from build123d import *

# Parameters (mm, degrees)
F0_W      = 203.2
F0_H      = 152.4
F2_DEPTH  = 152.4
F3_W      = 88.9
F3_H      = 139.7
F4_DEPTH  = 12.7
F5_R      = 6.35
F6_DEPTH  = 127
F1_R      = 44.45
F8_DEPTH  = 101.6
F9_R      = 5.08
F10_W     = 127
F10_H     = 139.7
F11_DEPTH = 101.6
F12_W     = 193.04
F12_H     = 142.24
F12_W_2   = 88.9
F12_H_2   = 139.7
F12_R     = 44.45
F12_R_2   = 6.35
F14_W     = 88.9
F14_H     = 139.7
F14_W_2   = 312.5441968441
F14_H_2   = 209.9168300629
F15_DEPTH = 29.21
F13_W     = 76.2
F13_H     = 127
F16_DEPTH = 152.4
F17_W     = 88.9
F17_H     = 127
F18_DEPTH = 253.619
F19_W     = 12.7
F19_H     = 38.596359849
F19_H_2   = 95.0815806389
F19_H_3   = 79.8769908249
F19_H_4   = 69.7309503555
F19_H_5   = 88.4333456159
F20_DEPTH = 6.35
F21_W     = 76.2
F21_H     = 12.7
F22_DEPTH = 6.35
F23_W     = 12.7
F23_H     = 76.2
F23_H_2   = 86.7299305499
F23_H_3   = 88.9
F24_DEPTH = 6.35
F25_W     = 12.7
F25_H     = 12.7
F25_H_2   = 12.4177324921
F25_H_3   = 127
F25_W_2   = 2.5730909735
F25_H_4   = 12.9822675079
F26_DEPTH = 12.7


with BuildPart() as f2:
    # F0 (on Front) → F2 (new body)
    with BuildSketch(Plane.XZ):
        Rectangle(F0_W, F0_H)
    extrude(amount=F2_DEPTH)

    # F3 (on Front) → F4 (cut)
    with BuildSketch(Plane.XZ):
        with Locations((-50.6012091197, -0.215793407)):
            Rectangle(F3_W, F3_H)
    extrude(amount=F4_DEPTH, mode=Mode.SUBTRACT)

    # F5 (on face) → F6 (cut)
    with BuildSketch(Plane(origin=(0, -12.7, 0), x_dir=(-1, 0, 0), z_dir=(0, 1, 0))):
        with Locations((19.2305770945, 52.8817098261)):
            Circle(F5_R)
        with Locations((19.2305770945, 31.2917098261)):
            Circle(F5_R)
        with Locations((19.2305770945, 9.7017098261)):
            Circle(F5_R)
        with Locations((19.2305770945, -11.8882901739)):
            Circle(F5_R)
        with Locations((19.2305770945, -33.4782901739)):
            Circle(F5_R)
        with Locations((19.2305770945, -55.0682901739)):
            Circle(F5_R)
        with Locations((40.8205770945, 52.8817098261)):
            Circle(F5_R)
        with Locations((40.8205770945, 31.2917098261)):
            Circle(F5_R)
        with Locations((40.8205770945, 9.7017098261)):
            Circle(F5_R)
        with Locations((40.8205770945, -11.8882901739)):
            Circle(F5_R)
        with Locations((40.8205770945, -33.4782901739)):
            Circle(F5_R)
        with Locations((40.8205770945, -55.0682901739)):
            Circle(F5_R)
        with Locations((62.4105770945, 52.8817098261)):
            Circle(F5_R)
        with Locations((62.4105770945, 31.2917098261)):
            Circle(F5_R)
        with Locations((62.4105770945, 9.7017098261)):
            Circle(F5_R)
        with Locations((62.4105770945, -11.8882901739)):
            Circle(F5_R)
        with Locations((62.4105770945, -33.4782901739)):
            Circle(F5_R)
        with Locations((62.4105770945, -55.0682901739)):
            Circle(F5_R)
        with Locations((84.0005770945, 52.8817098261)):
            Circle(F5_R)
        with Locations((84.0005770945, 31.2917098261)):
            Circle(F5_R)
        with Locations((84.0005770945, 9.7017098261)):
            Circle(F5_R)
        with Locations((84.0005770945, -11.8882901739)):
            Circle(F5_R)
        with Locations((84.0005770945, -33.4782901739)):
            Circle(F5_R)
        with Locations((84.0005770945, -55.0682901739)):
            Circle(F5_R)
    extrude(amount=-F6_DEPTH, mode=Mode.SUBTRACT)

    # F1 (on face) → F8 (cut)
    with BuildSketch(Plane.XZ):
        with Locations((48.0613298714, 0)):
            Circle(F1_R)
    extrude(amount=F8_DEPTH, mode=Mode.SUBTRACT)

    # F9
    f9_edges = [f2.edges().sort_by_distance(p)[0] for p in [
        (0, 0, 76.2),
        (101.6, 0, 0),
        (0, 0, -76.2),
        (-101.6, 0, 0),
        (-101.6, -76.2, -76.2),
        (101.6, -76.2, -76.2),
        (101.6, -76.2, 76.2),
        (-101.6, -76.2, 76.2),
    ]]
    fillet(f9_edges, radius=F9_R)

    # F10 (on face) → F11 (cut)
    with BuildSketch(Plane(origin=(-101.6, 0, 0), x_dir=(0, -1, 0), z_dir=(-1, 0, 0))):
        with Locations((76.9326984882, 0)):
            Rectangle(F10_W, F10_H)
    extrude(amount=-F11_DEPTH, mode=Mode.SUBTRACT)

    # F12 (on face) + F14 (on face) → F15 (cut)
    with BuildSketch(Plane(origin=(0, 0, 0), x_dir=(-1, 0, 0), z_dir=(0, 1, 0))):
        Rectangle(F12_W, F12_H)
        with Locations((50.6012091197, -0.215793407)):
            Rectangle(F12_W_2, F12_H_2, mode=Mode.SUBTRACT)
        with Locations((-48.0613298714, 0)):
            Circle(F12_R, mode=Mode.SUBTRACT)
        with Locations((-87.3994901776, 62.0860531926)):
            Circle(F12_R_2, mode=Mode.SUBTRACT)
    with BuildSketch(Plane(origin=(0, 0, 0), x_dir=(-1, 0, 0), z_dir=(0, 1, 0))):
        with Locations((50.6012091197, -0.215793407)):
            Rectangle(F14_W, F14_H)
        Rectangle(F14_W_2, F14_H_2)
    extrude(amount=-F15_DEPTH, mode=Mode.SUBTRACT)

    # F13 (on face) → F16 (cut)
    with BuildSketch(Plane(origin=(0, 0, -76.2), x_dir=(1, 0, 0), z_dir=(0, 0, -1))):
        with Locations((-52.4439588189, 78.7642598152)):
            Rectangle(F13_W, F13_H)
    extrude(amount=-F16_DEPTH, mode=Mode.SUBTRACT)

    # F17 (on Top) → F18 (cut, symmetric)
    with BuildSketch(Plane.XY):
        with Locations((40.8431477845, -78.819476068)):
            Rectangle(F17_W, F17_H)
    extrude(amount=F18_DEPTH, both=True, mode=Mode.SUBTRACT)

    # F19 (on face) → F20 (join)
    with BuildSketch(Plane.XY.offset(76.2)):
        with Locations((78.9431477845, -123.0212961435)):
            Rectangle(F19_W, F19_H)
        Polygon((59.8931477845, -142.319476068), (59.8931477845, -56.6326193511), (59.8931477845, -28.019476068), (47.1931477845, -28.019476068), (47.1931477845, -47.2378954291), (47.1931477845, -142.319476068), align=None)
        Polygon((72.5931477845, -142.319476068), (72.5931477845, -103.723116219), (72.5931477845, -56.6326193511), (59.8931477845, -56.6326193511), (59.8931477845, -142.319476068), align=None)
        with Locations((40.8431477845, -94.7786857486)):
            Rectangle(F19_W, F19_H_2)
        Polygon((21.7931477845, -62.4424852431), (21.7931477845, -142.319476068), (34.4931477845, -142.319476068), (34.4931477845, -47.2378954291), (34.4931477845, 16.430523932), (21.7931477845, 16.430523932), align=None)
        with Locations((15.4431477845, -102.3809806556)):
            Rectangle(F19_W, F19_H_3)
        with Locations((-20.6939588189, -107.3987846375)):
            Rectangle(F19_W, F19_H_4)
        Polygon((-39.7439588189, -53.8309141994), (-39.7439588189, -142.2642598152), (-27.0439588189, -142.2642598152), (-27.0439588189, -72.5333094597), (-27.0439588189, -27.9642598152), (-39.7439588189, -27.9642598152), align=None)
        with Locations((-46.0939588189, -98.0475870073)):
            Rectangle(F19_W, F19_H_5)
        Polygon((-65.1439588189, -40.6642598152), (-65.1439588189, -142.2642598152), (-52.4439588189, -142.2642598152), (-52.4439588189, -53.8309141994), (-52.4439588189, 10.1357401848), (-65.1439588189, 10.1357401848), align=None)
        Polygon((-77.8439588189, -91.4642598152), (-77.8439588189, -142.2642598152), (-65.1439588189, -142.2642598152), (-65.1439588189, -40.6642598152), (-77.8439588189, -40.6642598152), align=None)
        Polygon((-3.6068522155, -28.019476068), (-3.6068522155, -29.21), (-3.6068522155, -142.319476068), (9.0931477845, -142.319476068), (9.0931477845, -62.4424852431), (9.0931477845, -28.019476068), align=None)
    extrude(amount=-F20_DEPTH)

    # F21 (on face) → F22 (join)
    with BuildSketch(Plane(origin=(-101.6, 0, 0), x_dir=(0, -1, 0), z_dir=(-1, 0, 0))):
        Polygon((13.4326984882, -57.15), (13.4326984882, -69.85), (140.4326984882, -69.85), (140.4326984882, -57.15), (64.2326984882, -57.15), align=None)
        with Locations((102.3326984882, -50.8)):
            Rectangle(F21_W, F21_H)
        Polygon((26.1326984882, -25.4), (26.1326984882, -38.1), (140.4326984882, -38.1), (140.4326984882, -25.4), (64.2326984882, -25.4), align=None)
        with Locations((102.3326984882, -19.05)):
            Rectangle(F21_W, F21_H)
        Polygon((64.2326984882, -12.7), (140.4326984882, -12.7), (140.4326984882, 0), (41.91, 0), (41.91, -12.7), align=None)
        Polygon((41.91, 0), (140.4326984882, 0), (140.4326984882, 12.7), (38.8326984882, 12.7), (38.8326984882, 0), align=None)
        Polygon((13.4326984882, 31.75), (13.4326984882, 19.05), (140.4326984882, 19.05), (140.4326984882, 31.75), (26.1326984882, 31.75), align=None)
        Polygon((26.1326984882, 31.75), (140.4326984882, 31.75), (140.4326984882, 44.45), (64.2326984882, 44.45), (26.1326984882, 44.45), align=None)
        with Locations((102.3326984882, 50.8)):
            Rectangle(F21_W, F21_H)
        Polygon((64.2326984882, 57.15), (140.4326984882, 57.15), (140.4326984882, 69.85), (26.1326984882, 69.85), (26.1326984882, 57.15), align=None)
    extrude(amount=-F22_DEPTH)

    # F23 (on face) → F24 (join)
    with BuildSketch(Plane(origin=(0, 0, -76.2), x_dir=(1, 0, 0), z_dir=(0, 0, -1))):
        with Locations((78.9431477845, 104.219476068)):
            Rectangle(F23_W, F23_H)
        with Locations((2.7431477845, 98.9545107931)):
            Rectangle(F23_W, F23_H_2)
        with Locations((-20.6939588189, 97.8142598152)):
            Rectangle(F23_W, F23_H_3)
        Polygon((72.5931477845, 28.019476068), (72.5931477845, 66.119476068), (72.5931477845, 142.319476068), (59.8931477845, 142.319476068), (59.8931477845, 28.019476068), align=None)
        Polygon((59.8931477845, 28.019476068), (59.8931477845, 142.319476068), (47.1931477845, 142.319476068), (47.1931477845, 53.419476068), (47.1931477845, 15.319476068), (59.8931477845, 15.319476068), align=None)
        with Locations((40.8431477845, 97.869476068)):
            Rectangle(F23_W, F23_H_3)
        Polygon((34.4931477845, 53.419476068), (34.4931477845, 142.319476068), (21.7931477845, 142.319476068), (21.7931477845, 40.719476068), (21.7931477845, 28.019476068), (34.4931477845, 28.019476068), align=None)
        Polygon((21.7931477845, 40.719476068), (21.7931477845, 142.319476068), (9.0931477845, 142.319476068), (9.0931477845, 55.5895455182), (9.0931477845, 40.719476068), align=None)
        Polygon((-27.0439588189, 142.2642598152), (-39.7439588189, 142.2642598152), (-39.7439588189, 34.2246964574), (-27.0439588189, 34.2246964574), (-27.0439588189, 53.3642598152), align=None)
        Polygon((-39.7439588189, 142.2642598152), (-52.4439588189, 142.2642598152), (-52.4439588189, 27.9642598152), (-39.7439588189, 27.9642598152), (-39.7439588189, 34.2246964574), align=None)
        Polygon((-52.4439588189, 142.2642598152), (-65.1439588189, 142.2642598152), (-65.1439588189, 66.0642598152), (-65.1439588189, 2.5642598152), (-52.4439588189, 2.5642598152), (-52.4439588189, 27.9642598152), align=None)
        with Locations((-71.4939588189, 104.1642598152)):
            Rectangle(F23_W, F23_H)
        Polygon((-90.5439588189, 142.2642598152), (-90.5439588189, 29.21), (-90.5439588189, 27.9642598152), (-77.8439588189, 27.9642598152), (-77.8439588189, 66.0642598152), (-77.8439588189, 142.2642598152), align=None)
    extrude(amount=-F24_DEPTH)

    # F25 (on face) → F26 (join)
    with BuildSketch(Plane.XZ.offset(152.4)):
        Polygon((85.4586139321, 64.0224360317), (61.2050529242, 64.0224360317), (48.5050529242, 64.0224360317), (7.57732118, 64.0224360317), (-5.12267882, 64.0224360317), (-26.6723212183, 64.0224360317), (-39.3723212183, 64.0224360317), (-102.4682950944, 64.0224360317), (-102.4682950944, 44.3732525826), (-89.7682950944, 44.3732525826), (-89.7682950944, 31.6732525826), (-102.4682950944, 31.6732525826), (-102.4682950944, -25.3421988666), (-89.7682950944, -25.3421988666), (-89.7682950944, -38.0421988666), (-102.4682950944, -38.0421988666), (-102.4682950944, -62.9775639683), (-89.4405841827, -62.9775639683), (-76.7405841827, -62.9775639683), (-52.6970252395, -62.9775639683), (-39.9970252395, -62.9775639683), (22.5620511919, -62.9775639683), (35.2620511919, -62.9775639683), (59.3553744256, -62.9775639683), (72.0553744256, -62.9775639683), (85.4586139321, -62.9775639683), align=None)
        with Locations((54.8550529242, 70.3724360317)):
            Rectangle(F25_W, F25_H)
        with Locations((91.8086139321, 70.2313022777)):
            Rectangle(F25_W, F25_H_2)
        with Locations((91.8086139321, 0.5224360317)):
            Rectangle(F25_W, F25_H_3)
        with Locations((1.22732118, 70.3724360317)):
            Rectangle(F25_W, F25_H)
        with Locations((99.4451594189, 0.5224360317)):
            Rectangle(F25_W_2, F25_H_3)
        with Locations((91.8086139321, -69.4686977223)):
            Rectangle(F25_W, F25_H_4)
        with Locations((65.7053744256, -69.3275639683)):
            Rectangle(F25_W, F25_H)
        with Locations((-33.0223212183, 70.3724360317)):
            Rectangle(F25_W, F25_H)
        with Locations((28.9120511919, -69.3275639683)):
            Rectangle(F25_W, F25_H)
        with Locations((-96.1182950944, 38.0232525826)):
            Rectangle(F25_W, F25_H)
        with Locations((-46.3470252395, -69.3275639683)):
            Rectangle(F25_W, F25_H)
        with Locations((-96.1182950944, -31.6921988666)):
            Rectangle(F25_W, F25_H)
        with Locations((-83.0905841827, -69.3275639683)):
            Rectangle(F25_W, F25_H)
    extrude(amount=F26_DEPTH)


solid = f2.part
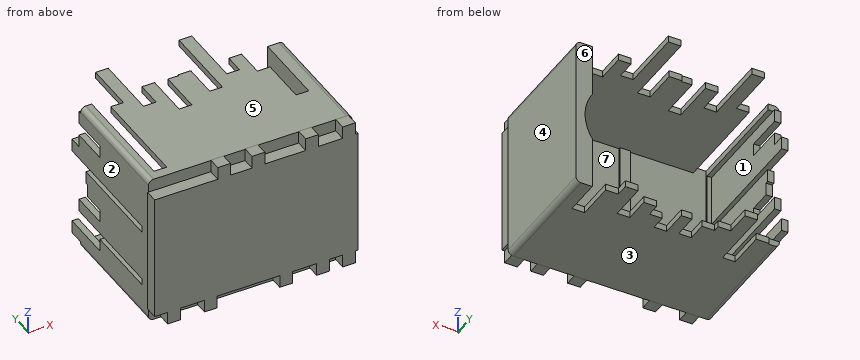
Geometry check sheet. Reference: the model listing, model coordinates, mm. Face numbers are marked on the shaded views. A direction names the side the tool comes from. Give positions to 0.01 mm unless a question says otherwise; leave off trailing zeros. Order: outer loops, then holes, each group sorted by start corner. A loop starts at its lowest first (then second) coordinate and runs counter-clockwise, first axis right, second up.
1) Cross-section at B-B (y = -135.5). Record the boundary of the cut face in (x, z).
Results are:
outline: (-101.6, -71.12) arc R5.08 ccw to (-96.52, -76.2) - (96.52, -76.2) arc R5.08 ccw to (101.6, -71.12) - (101.6, 71.12) arc R5.08 ccw to (96.52, 76.2) - (-77.84, 76.2) - (-77.84, 69.85) - (85.29, 69.85) - (85.29, -69.85) - (-95.25, -69.85) - (-95.25, -44.45) - (-101.6, -44.45) - close; (-101.6, -38.1) - (-95.25, -38.1) - (-95.25, 12.7) - (-101.6, 12.7) - close; (-101.6, 19.05) - (-95.25, 19.05) - (-95.25, 69.85) - (-90.54, 69.85) - (-90.54, 76.2) - (-96.52, 76.2) arc R5.08 ccw to (-101.6, 71.12) - close
2) Material ranges on probe 1 along X at (y, z) = (-65, 70.5); probe 2 along Z at (x, y) = (24, -87); probe 3 along X at (y, z) = (-107, 0.5), recorded low to high.
Results are:
probe 1: x = -101.6 to -90.54, -77.84 to -27.04, -14.34 to 72.59, 85.29 to 101.6
probe 2: z = -76.2 to -69.85, 69.85 to 76.2
probe 3: x = -101.6 to -95.25, 85.29 to 101.6
3) Cross-section at C-C (x = 56). Record the boundary of the cut face in (y, z).
Results are:
outline: (-165.1, -62.98) - (-152.4, -62.98) - (-152.4, -76.2) - (-15.32, -76.2) - (-15.32, -69.85) - (-142.32, -69.85) - (-142.32, 69.85) - (-28.02, 69.85) - (-28.02, 76.2) - (-152.4, 76.2) - (-152.4, 76.72) - (-165.1, 76.72) - close
4) Tool access check on the marked faces 5, 6 and 7. Record the directions out of +Z, -Z, +X, -X, +Y, -Y that give a thin tool (end or side, any length) a straight path to the whole face; none if there is none.
Results are:
face 5: +Z, +X, -X, +Y
face 6: +Z, -Z, +X, +Y
face 7: +Y
5) Draft check along X on the marked faces 1, 2, 3 and 4. Enter one of: released by +X, released by -X, zero draft, split by the parting line, or undercut.
Results are:
face 1: undercut
face 2: released by -X
face 3: zero draft
face 4: released by +X
6) Gauge pin test, flat ends, axial feed: pin 1 (5 mm diameter, centred on x = -97.5, z = 49, fed in from +Y); pin 2 (6 mm diameter, centred on x = -66.5, z = -19.5, fed in from +Y); pin 3 (13.5 mm diameter, centred on y = -156, z = 71, fed in from -X); pin 4 (5 mm diameter, centred on x = -99, y = -72, fed in from -Z). Record the tip position at first contact, or that the pin passes through.
Results are:
pin 1: stops at y = -64.23
pin 2: stops at y = -142.26
pin 3: stops at x = -101.6
pin 4: stops at z = -76.2
7) Cross-section at A-A (y = -21). Record the boundary of the cut face in (x, z), then the cut area to 3 significant figures.
Results are:
outline: (-101.6, -69.85) - (-95.25, -69.85) - (-95.25, -57.15) - (-101.6, -57.15) - close; (-101.6, 19.05) - (-95.25, 19.05) - (-95.25, 31.75) - (-101.6, 31.75) - close; (-65.14, -76.2) - (-52.44, -76.2) - (-52.44, -69.85) - (-65.14, -69.85) - close; (-65.14, 69.85) - (-52.44, 69.85) - (-52.44, 76.2) - (-65.14, 76.2) - close; (21.79, 69.85) - (34.49, 69.85) - (34.49, 76.2) - (21.79, 76.2) - close; (47.19, -76.2) - (59.89, -76.2) - (59.89, -69.85) - (47.19, -69.85) - close
area: 484 mm2
8) Cross-section at D-D (z = 40.5). Record the boundary of the cut face in (x, y), then the cut area to 3 significant figures.
Results are:
outline: (-102.47, -165.1) - (100.73, -165.1) - (100.73, -152.4) - (101.6, -152.4) - (101.6, -29.21) - (85.29, -29.21) - (85.29, -142.32) - (-3.61, -142.32) - (-3.61, -140.43) - (-14.34, -140.43) - (-14.34, -142.26) - (-90.54, -142.26) - (-90.54, -140.43) - (-95.25, -140.43) - (-95.25, -26.13) - (-101.6, -26.13) - (-101.6, -152.4) - (-102.47, -152.4) - close
area: 7,240 mm2
